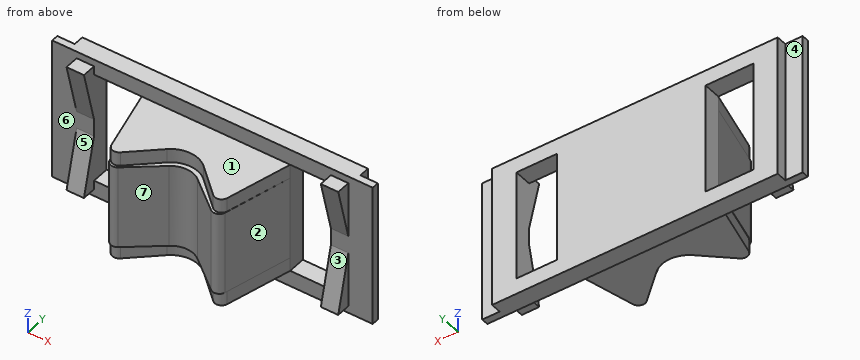
from build123d import *

# Parameters (mm, degrees)
SKETCH_1_W                = 75.557626564
SKETCH_1_H                = 3.901331086
EXTRUDE_1_DEPTH           = 25
SKETCH_1_H_2              = 4
EXTRUDE_1_2_DEPTH         = 25
CUT_EXTRUDE_15_DEPTH      = 32
SKETCH_1_6_W              = 75.557626564
SKETCH_1_6_H              = 24
EXTRUDE_5_DEPTH           = 25
CUT_EXTRUDE_16_DEPTH      = 153.500220667
CUT_EXTRUDE_16_DEPTH_BACK = 153.500220667
SKETCH_3_R                = 6.5
FILLET_2_R                = 2
FILLET_3_R                = 2
EXTRUDE_6_DEPTH           = 5
EXTRUDE_6_2_DEPTH         = 5
EXTRUDE_7_DEPTH           = 5
EXTRUDE_7_2_DEPTH         = 5
SKETCH_6_W                = 82
SKETCH_6_H                = 41
SKETCH_6_W_2              = 13.693142479
SKETCH_6_H_2              = 31.901331086
SKETCH_6_W_3              = 11.689861707
EXTRUDE_8_DEPTH           = 5
SKETCH_7_W                = 5
SKETCH_7_H                = 41
EXTRUDE_9_DEPTH           = 2
CUT_EXTRUDE_17_DEPTH      = 163.242088223
CUT_EXTRUDE_17_DEPTH_BACK = 163.242088223


with BuildPart() as part:
    # Sketch 1 → Extrude 1 (new body)
    with BuildSketch(Plane(origin=(0, 102.001425994, 0), x_dir=(1, 0, 0), z_dir=(0, 1, 0))):
        with Locations((68.52058233, -72.602036932)):
            Rectangle(SKETCH_1_W, SKETCH_1_H)
    extrude(amount=-EXTRUDE_1_DEPTH)


with BuildPart() as body_2:
    # Sketch 1 → Extrude 1 2 (new body)
    with BuildSketch(Plane(origin=(0, 102.001425994, 0), x_dir=(1, 0, 0), z_dir=(0, 1, 0))):
        with Locations((68.52058233, -100.552702475)):
            Rectangle(SKETCH_1_W, SKETCH_1_H_2)
    extrude(amount=-EXTRUDE_1_2_DEPTH)


with BuildPart() as cut_extrude_15_tool:
    # Sketch 2 → Cut-Extrude 15 (new body)
    with BuildSketch(Plane.XY.offset(102.552702475)):
        with BuildLine():
            Line((63.510266919, 89.850934142), (52.937126115, 80.258094246))
            Line((52.937126115, 80.258094246), (47.434911527, 102.001425994))
            Line((47.434911527, 102.001425994), (30.741769048, 102.001425994))
            Line((30.741769048, 102.001425994), (30.741769048, 77.001425994))
            Line((30.741769048, 77.001425994), (106.299395612, 77.001425994))
            Line((106.299395612, 77.001425994), (106.299395612, 102.001425994))
            Line((106.299395612, 102.001425994), (90.051907341, 102.001425994))
            Line((90.051907341, 102.001425994), (84.547557962, 80.262935973))
            Line((84.547557962, 80.262935973), (73.973273177, 89.850934142))
            ThreePointArc((73.973273177, 89.850934142), (68.741770048, 91.84906096), (63.510266919, 89.850934142))
        make_face()
    extrude(amount=-CUT_EXTRUDE_15_DEPTH)


with BuildPart() as part_1:
    add(part.part)

    # Cut-Extrude 15: cut by cut_extrude_15_tool
    add(cut_extrude_15_tool.part, mode=Mode.SUBTRACT)



with BuildPart() as body_2_1:
    add(body_2.part)

    # Cut-Extrude 15: cut by cut_extrude_15_tool
    add(cut_extrude_15_tool.part, mode=Mode.SUBTRACT)


with BuildPart() as part_2:
    add(part_1.part)

    add(body_2_1.part)  # Extrude 5 merges body 2
    # Sketch 1_6 → Extrude 5 (add)
    with BuildSketch(Plane(origin=(0, 102.001425994, 0), x_dir=(1, 0, 0), z_dir=(0, 1, 0))):
        with Locations((68.52058233, -86.552702475)):
            Rectangle(SKETCH_1_6_W, SKETCH_1_6_H)
    extrude(amount=-EXTRUDE_5_DEPTH)

    # Sketch 3 → Cut-Extrude 16 (cut, two sides: drawn at the far end of the back side and taken through both)
    with BuildSketch(Plane.XY.offset(110.052702475).offset(-CUT_EXTRUDE_16_DEPTH_BACK)):
        with BuildLine():
            Line((52.937126115, 79.748220071), (47.431470764, 102.001425994))
            Line((47.431470764, 102.001425994), (30.73376132, 102.001425994))
            Line((30.73376132, 102.001425994), (30.741769048, 77.001425994))
            Line((30.741769048, 77.001425994), (88.549097609, 77.001425994))
            ThreePointArc((88.549097609, 77.001425994), (92.13390173, 85.931402357), (99.789402086, 80.101426994))
            ThreePointArc((99.789402086, 80.101426994), (99.571745411, 78.493558676), (98.934442488, 77.001425994))
            Line((98.934442488, 77.001425994), (106.299395612, 77.001425994))
            Line((106.299395612, 77.001425994), (106.299395612, 102.001425994))
            Line((106.299395612, 102.001425994), (90.051907341, 102.001425994))
            Line((90.051907341, 102.001425994), (84.489905965, 79.748220071))
            Line((84.489905965, 79.748220071), (72.796657252, 89.081573622))
            ThreePointArc((72.796657252, 89.081573622), (74.598679081, 86.82040138), (75.241770048, 84.001426994))
            ThreePointArc((75.241770048, 84.001426994), (65.922795662, 78.144517962), (64.686882844, 89.081573622))
            Line((64.686882844, 89.081573622), (52.937126115, 79.748220071))
        make_face()
        with Locations((68.741770048, 84.001426994)):
            Circle(SKETCH_3_R)
    extrude(amount=CUT_EXTRUDE_16_DEPTH + CUT_EXTRUDE_16_DEPTH_BACK, mode=Mode.SUBTRACT)


with BuildPart() as cut_extrude_16_piece_1:
    # of the separate pieces the step leaves, piece 1, a body of its own (cut_extrude_16_pieces)
    add(part_2.part.solids().sort_by_distance((47.431470764, 102.001425994, 74.552702475))[0])

    # Fillet 2
    fillet_2_edges = [cut_extrude_16_piece_1.edges().sort_by_distance(p)[0] for p in [
        (52.937126115, 80.258094246, 72.602036932),
        (84.547557962, 80.262935973, 72.602036932),
        (84.547557962, 80.262935973, 100.552702475),
        (52.937126115, 80.258094246, 100.552702475),
    ]]
    fillet(fillet_2_edges, radius=FILLET_2_R)

    # Fillet 3
    fillet_3_edges = [cut_extrude_16_piece_1.edges().sort_by_distance(p)[0] for p in [
        (52.937126115, 79.748220071, 86.552702475),
        (84.489905965, 79.748220071, 86.552702475),
    ]]
    fillet(fillet_3_edges, radius=FILLET_3_R)



with BuildPart() as cut_extrude_16_piece_2:
    # of the separate pieces the step leaves, piece 2, a body of its own (cut_extrude_16_pieces)
    add(part_2.part.solids().sort_by_distance((99.789402086, 80.101426994, 74.552702475))[0])

    # Sketch 3_3 → Cut-Extrude 17 (cut, two sides: drawn at the far end of the back side and taken through both)
    with BuildSketch(Plane.XY.offset(110.052702475).offset(-CUT_EXTRUDE_17_DEPTH_BACK)):
        with BuildLine():
            ThreePointArc((99.789402086, 80.101426994), (92.13390173, 85.931402357), (88.549097609, 77.001425994))
            Line((88.549097609, 77.001425994), (98.934442488, 77.001425994))
            ThreePointArc((98.934442488, 77.001425994), (99.571745411, 78.493558676), (99.789402086, 80.101426994))
        make_face()
        with BuildLine():
            Line((98.934442488, 77.001425994), (88.549097609, 77.001425994))
            ThreePointArc((88.549097609, 77.001425994), (93.741770048, 74.053794956), (98.934442488, 77.001425994))
        make_face()
    extrude(amount=CUT_EXTRUDE_17_DEPTH + CUT_EXTRUDE_17_DEPTH_BACK, mode=Mode.SUBTRACT)


with BuildPart() as body_3:
    # Sketch 4 → Extrude 6 (new body)
    with BuildSketch(Plane(origin=(28.741769048, 0, 0), x_dir=(0, 0, -1), z_dir=(1, 0, 0))):
        Polygon((-105.052702475, 102.001425994), (-105.052702475, 98.001425994), (-89.052702475, 102.001425994), align=None)
    extrude(amount=EXTRUDE_6_DEPTH)


with BuildPart() as body_4:
    # Sketch 4 → Extrude 6 2 (new body)
    with BuildSketch(Plane(origin=(28.741769048, 0, 0), x_dir=(0, 0, -1), z_dir=(1, 0, 0))):
        Polygon((-68.052702475, 102.001425994), (-68.052702475, 98.001425994), (-84.052702475, 102.001425994), align=None)
    extrude(amount=EXTRUDE_6_2_DEPTH)


with BuildPart() as body_5:
    # Sketch 5 → Extrude 7 (new body)
    with BuildSketch(Plane.ZY.offset(-106.741769048)):
        Polygon((105.052702475, 102.001425994), (105.052702475, 98.001425994), (89.052702475, 102.001425994), align=None)
    extrude(amount=EXTRUDE_7_DEPTH)


with BuildPart() as body_6:
    # Sketch 5 → Extrude 7 2 (new body)
    with BuildSketch(Plane.ZY.offset(-106.741769048)):
        Polygon((68.052702475, 102.001425994), (84.052702475, 102.001425994), (68.052702475, 98.001425994), align=None)
    extrude(amount=EXTRUDE_7_2_DEPTH)


with BuildPart() as cut_extrude_16_piece_1_1:
    add(cut_extrude_16_piece_1.part)

    add(body_3.part)  # Extrude 8 merges body 3

    add(body_4.part)  # Extrude 8 merges body 4

    add(body_5.part)  # Extrude 8 merges body 5

    add(body_6.part)  # Extrude 8 merges body 6
    # Sketch 6 → Extrude 8 (add)
    with BuildSketch(Plane(origin=(0, 102.001425994, 0), x_dir=(1, 0, 0), z_dir=(0, 1, 0))):
        with Locations((67.741769048, -86.552702475)):
            Rectangle(SKETCH_6_W, SKETCH_6_H)
        with Locations((40.588340288, -86.602036932)):
            Rectangle(SKETCH_6_W_2, SKETCH_6_H_2, mode=Mode.SUBTRACT)
        with Locations((95.896838195, -86.602036932)):
            Rectangle(SKETCH_6_W_3, SKETCH_6_H_2, mode=Mode.SUBTRACT)
    extrude(amount=EXTRUDE_8_DEPTH)

    # Sketch 7 → Extrude 9 (add)
    with BuildSketch(Plane(origin=(0, 102.001425994, 0), x_dir=(1, 0, 0), z_dir=(0, 1, 0))):
        with Locations((24.241769048, -86.552702475)):
            Rectangle(SKETCH_7_W, SKETCH_7_H)
        with Locations((111.241769048, -86.552702475)):
            Rectangle(SKETCH_7_W, SKETCH_7_H)
    extrude(amount=EXTRUDE_9_DEPTH)


solid = cut_extrude_16_piece_1_1.part
For this review, take the finished solid that the model builds, in its own axes (mm). Face numbers are marked on the shaded views. A direction names the side the tool comes from. Coordinates: 2 decimals unless noted, no trailing zeros. Order: outer loops, then holes, each group sorted by start corner. A loop starts at its lowest first (then second) coordinate and runs counter-clockwise, first axis right, second up. Notation, with made-up numbers: (32, -38) -> (78, -38) arc R38 cw to (78, 0) -> close; hole circle Ø2 at (-19.75, 1). An arc over 180 degrees is marked (long way). Return JSON: item names as keys, results as strings.
1. The part is to be moulded in two halves that separate along Z. For the marked faces 1, 2 and 3, say which applies: +Z half, -Z half, draft (parallel to the pull), parting line (faces both ways), or undercut.
Answer block:
{"face 1": "+Z half", "face 2": "draft", "face 3": "undercut"}
2. Machinability: for the marked faces 4, 5, 6 and 7, which of the approach directions +Z, -Z, +X, -X, +Y, -Y give a long, thin tool a straight path to every point of the face, cutting with its end or side? Answer none if there is none.
Answer block:
{"face 4": "+Z, -Z, -X, +Y", "face 5": "-X, -Y", "face 6": "-Y", "face 7": "+Z, -Z, -Y"}
3. We need section D-D on y = 87. Write out the cut boundary in (x, z).
Answer block:
{"outline": "(51.14, 74.55) -> (51.23, 74.55) -> (51.23, 70.65) -> (60.37, 70.65) -> (60.37, 74.55) -> (62.07, 74.55) -> (62.07, 98.55) -> (60.37, 98.55) -> (60.37, 102.55) -> (51.23, 102.55) -> (51.23, 98.55) -> (51.14, 98.55) -> close; (75.4, 74.55) -> (77.12, 74.55) -> (77.12, 70.65) -> (86.25, 70.65) -> (86.25, 74.55) -> (86.3, 74.55) -> (86.3, 98.55) -> (86.25, 98.55) -> (86.25, 102.55) -> (77.12, 102.55) -> (77.12, 98.55) -> (75.4, 98.55) -> close"}
4. For pin 1 Ø1 at (y, z) = (89, 95) entering from +X; pin 2 Ø2.5 at (x, z) = (112, 78.5) entering from +Y; pin 3 Ø4 at (y, z) = (84, 87) entering from -X, all flat-tipped, find the tip position at first contact; note any pin that passes through.
Answer block:
{"pin 1": "x = 86.93", "pin 2": "y = 104", "pin 3": "x = 51.39"}
5. We need section B-B on x = 104. Write out the cut boundary in (y, z), and give its area (3 significant figures).
Answer block:
{"outline": "(98, 68.05) -> (102, 68.05) -> (102, 66.05) -> (107, 66.05) -> (107, 107.05) -> (102, 107.05) -> (102, 105.05) -> (98, 105.05) -> (102, 89.05) -> (102, 84.05) -> close", "area": "269 mm²"}
6. We need section A-A on z = 85.5. State how many separate pieces and enclosed holes the cut face has, and give its area (3 significant figures).
Answer block:
{"separate pieces": "3", "enclosed holes": "0", "area": "931 mm²"}
7. For line 1 (X direction, y = 102.25, z = 72.5); line 2 (X direction, y = 104.5, z = 91); line 3 (Z direction, x = 40.5, y = 104.75), list the stretches that pass through material, from the lowest coordinate up. Write a range as from..to.
Answer block:
{"line 1": "21.74..33.74, 47.43..90.05, 101.74..113.74", "line 2": "26.74..33.74, 47.43..90.05, 101.74..108.74", "line 3": "66.05..70.65, 102.55..107.05"}
